The figure shows three views and two pictorial views of one solid part (mm, origin at its lowest corner). Answer the questions. A direction names the side the tool comes from. Give positions to 0.01 mm unless a question says otherwise; leave off trailing zeros. Write each loop counter-clockwise with the first axis right and the second up, starting at its lowest first coordinate (ties: lowest second). Pieces come first, ordered by that corner, then holes. Notation, with made-up numbers: (-26.5, 49.25) - (12.5, 49.25) arc R12 cw to (12.5, 61.25) - close; hole circle Ø1 at (64, 85.5). An arc over 180 degrees is marked (long way). Answer as CSV lines item,"result". Start each with the question number.
(1) For the marked faces 1 and 2, determine the directions among +Z, -Z, +X, -X, +Y, -Y from which every point of the face is accessible in a straight line to the end or side of a thin tool.
(2) For a pull along Y with two mould halves and no side action, classify the marked faces 3, 4 and 5 as pulls with the +Y half, pulls with the -Y half, needs draft (parallel to the pull), parting line crosses it, or undercut.
(3) Find section C-C (x = 7.5). Write down the section's boundary in (y, z).
(4) Each of these flat-tipped pins is pushed along its axis until it touches: pin 1 Ø2 at (x, z) = (7.5, 3) entering from +Y; pin 2 Ø8 at (x, y) = (13, 8.5) entering from +Z; pin 3 Ø3 at (x, y) = (8, 12) entering from -Z. Where does it stop, or does it pass through?
(5) Straight lines are drawn through the part: probe 1 along X at (y, z) = (3.65, 3); probe 2 along X at (y, z) = (11, 4.25); probe 3 along Y at (x, z) = (10.25, 5). For each, find the intervals that lie inside material, in ascending order.
(6) Find section B-B (y = 15). Write down the section's boundary in (x, z).
(7) Find section D-D (x = 9.25). Write down the section's boundary in (y, z), then the cut area to 3 significant figures.
(8) Find section A-A (z = 3). Write down the section's boundary in (x, y).
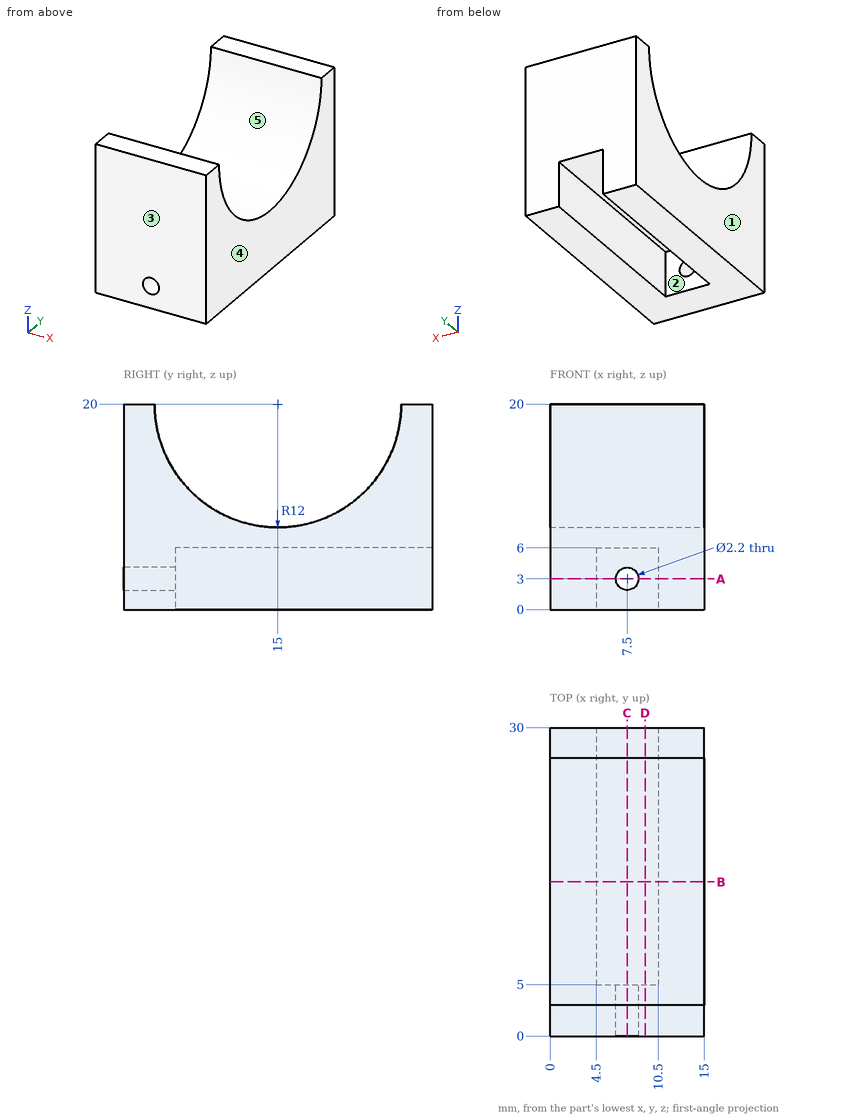
Result set:
1,face 1,"+Z, -Z, -X, +Y, -Y"
1,face 2,"-Z, +Y"
2,face 3,"pulls with the -Y half"
2,face 4,"needs draft"
2,face 5,"undercut"
3,outline,"(0, 0) - (5, 0) - (5, 1.9) - (0, 1.9) - close; (0, 4.1) - (5, 4.1) - (5, 6) - (30, 6) - (30, 20) - (27, 20) arc R12 cw to (3, 20) - (0, 20) - close"
4,pin 1,"through"
4,pin 2,"z = 14.19"
4,pin 3,"z = 6"
5,probe 1,"0 to 6.4, 8.6 to 15"
5,probe 2,"0 to 4.5, 10.5 to 15"
5,probe 3,"0 to 5"
6,outline,"(0, 0) - (4.5, 0) - (4.5, 6) - (10.5, 6) - (10.5, 0) - (15, 0) - (15, 8) - (0, 8) - close"
7,outline,"(0, 0) - (5, 0) - (5, 6) - (30, 6) - (30, 20) - (27, 20) arc R12 cw to (3, 20) - (0, 20) - close"
7,area,"224 mm^2"
8,outline,"(0, 0) - (6.4, 0) - (6.4, 5) - (4.5, 5) - (4.5, 30) - (0, 30) - close; (8.6, 0) - (15, 0) - (15, 30) - (10.5, 30) - (10.5, 5) - (8.6, 5) - close"
